from build123d import *

# Parameters (mm, degrees)
DODANIE_WYCI_GNI_CIE1_DEPTH = 5
OTW_R_POD_RUB_M51_D         = 5.5
OTW_R_POD_RUB_M51_DEPTH     = 14
OTW_R_POD_RUB_M51_TIP       = 1.652366702
OTW_R_POD_RUB_M52_D         = 5.5
OTW_R_POD_RUB_M52_DEPTH     = 14
OTW_R_POD_RUB_M52_TIP       = 1.652366702


with BuildPart() as part:
    # Szkic1 → Dodanie-wyciągnięcie1 (new body)
    with BuildSketch(Plane(origin=(1037.6, 0, 0), x_dir=(0, 0, -1), z_dir=(1, 0, 0))):
        with BuildLine():
            Line((-892.51, 75), (-632.51, 75))
            ThreePointArc((-632.51, 75), (-625.438932188, 72.071067812), (-622.51, 65))
            Line((-622.51, 65), (-622.51, -65))
            ThreePointArc((-622.51, -65), (-625.438932188, -72.071067812), (-632.51, -75))
            Line((-632.51, -75), (-892.51, -75))
            ThreePointArc((-892.51, -75), (-899.581067812, -72.071067812), (-902.51, -65))
            Line((-902.51, -65), (-902.51, 65))
            ThreePointArc((-902.51, 65), (-899.581067812, 72.071067812), (-892.51, 75))
        make_face()
    extrude(amount=-DODANIE_WYCI_GNI_CIE1_DEPTH)

    # Otwór pod śrubę M51
    with Locations(Plane.ZY.offset(-1032.6)):
        with Locations((634.12, 45), (634.12, -45)):
            Hole(OTW_R_POD_RUB_M51_D / 2, depth=OTW_R_POD_RUB_M51_DEPTH)
            with Locations((0, 0, -(OTW_R_POD_RUB_M51_DEPTH + OTW_R_POD_RUB_M51_TIP / 2))):  # 118° drill point
                Cone(0, OTW_R_POD_RUB_M51_D / 2, OTW_R_POD_RUB_M51_TIP, mode=Mode.SUBTRACT)

    # Otwór pod śrubę M52
    with Locations(Plane.ZY.offset(-1032.6)):
        with Locations((837.51, 45), (837.51, -45)):
            Hole(OTW_R_POD_RUB_M52_D / 2, depth=OTW_R_POD_RUB_M52_DEPTH)
            with Locations((0, 0, -(OTW_R_POD_RUB_M52_DEPTH + OTW_R_POD_RUB_M52_TIP / 2))):  # 118° drill point
                Cone(0, OTW_R_POD_RUB_M52_D / 2, OTW_R_POD_RUB_M52_TIP, mode=Mode.SUBTRACT)


solid = part.part
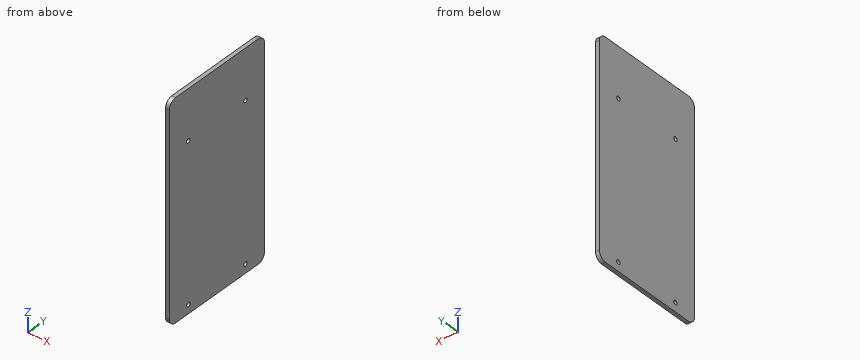
Geometry check sheet. Reference: the model listing, model coordinates, mm. Give positions to 0.01 mm unless a question says otherwise; leave off trailing zeros. Write each loop counter-clockwise with the first axis right and the second up, starting at its lowest first coordinate (ties: lowest second). Pieces come first, ordered by that corner, then holes. Notation, with made-up numbers: (64.25, 71.5) - (120.25, 71.5) arc R35 ccw to (120.25, 103.5) - close; hole circle Ø9 at (-35, 48.25). An arc over 180 degrees is marked (long way). Put each result on its own line as item: value.
1. Sectioned sample at A-A, the plane z = 837.51. Enter the section's corners in (x, y).
Ans:
outline: (1032.6, -75) - (1037.6, -75) - (1037.6, -47.75) - (1032.6, -47.75) - close; (1032.6, -42.25) - (1037.6, -42.25) - (1037.6, 42.25) - (1032.6, 42.25) - close; (1032.6, 47.75) - (1037.6, 47.75) - (1037.6, 75) - (1032.6, 75) - close
2. Thickness scan on line 1 (Y direction, x = 1035.65, z = 634.12); line 2 (Z direction, x = 1037.1, y = -46). Record the ranges inside material, lowest first.
Ans:
line 1: y = -75 to -47.75, -42.25 to 42.25, 47.75 to 75
line 2: z = 622.51 to 631.56, 636.68 to 834.95, 840.07 to 902.51
3. Sectioned sample at B-B, the plane y = 45. Enter the section's corners in (x, z).
Ans:
outline: (1032.6, 622.51) - (1037.6, 622.51) - (1037.6, 631.37) - (1032.6, 631.37) - close; (1032.6, 636.87) - (1037.6, 636.87) - (1037.6, 834.76) - (1032.6, 834.76) - close; (1032.6, 840.26) - (1037.6, 840.26) - (1037.6, 902.51) - (1032.6, 902.51) - close
4. Go/stop test with flat-tipped pins: pin 1 (7 mm diameter, centred on y = -45, z = 634.12, fed in from -X); pin 2 (4.5 mm diameter, centred on y = 45, z = 837.51, fed in from -X). Record where each tip stops, or that it passes through.
Ans:
pin 1: stops at x = 1032.6
pin 2: passes through
